Design review of the part shown in the three views and the two pictorial views. Dimensions are in mm from the part's minimum x, y and z. A direction names the side the tool comes from. Round coordinates to 2 decimals unless told otherwise and drop trailing zeros. Write each loop counter-clockwise with the first axis right and the second up, starting at its lowest first coordinate (ties: lowest second). Pieces come first, ordered by that corner, then holes. Notation, with made-up numbers: (45, 89.5) -> (78, 89.5) arc R30 ccw to (78, 118.5) -> close; hole circle Ø2 at (-29.75, 29). An arc over 180 degrees is marked (long way). Return JSON: item names as keys, results as strings. Group by question number.
1. For line 1 along Y through (x, z) = (11.5, 1.75); line 2 along X through (y, z) = (10.25, 6); line 3 along Z through (x, y) = (7, 7), list the stretches that pass through material, from the lowest coordinate up. Write a range as from..to.
2. Mouldability with a two-part tool opening along Y and no side actions: class the marked faces 1, 2 and 3 as pulls with the +Y half, pulls with the -Y half, needs draft (parallel to the pull), parting line crosses it, or undercut.
3. Clearance check with flat-ended pins moving along their axes: P1, Ø6.5, axis at y = 7, z = 6, coming from the +X side; P2, Ø2.5, axis at x = 6.5, z = 5, coming from the -Y side; P3, Ø0.6, axis at y = 13.5, z = 16.5, coming from the +X side. State where each tip first meets the part, or that it passes through.
4. Take a section at B-B, the plane z = 5.25. Write out the cut boundary in (x, y), then the cut area to 3 significant figures.
5. Take a section at A-A, the plane z = 1.5. Write out the cut boundary in (x, y).
6. Take a section at C-C, the plane x = 11.5. Give the number of separate pieces and of enclosed holes in the cut face, then the cut area to 3 significant figures.
7. Tool access review of the marked faces 4, 5 and 6: name each direction out of +Z, -Z, +X, -X, +Y, -Y from which nothing blocks a thin tool from reaching the whole face with its end or side.
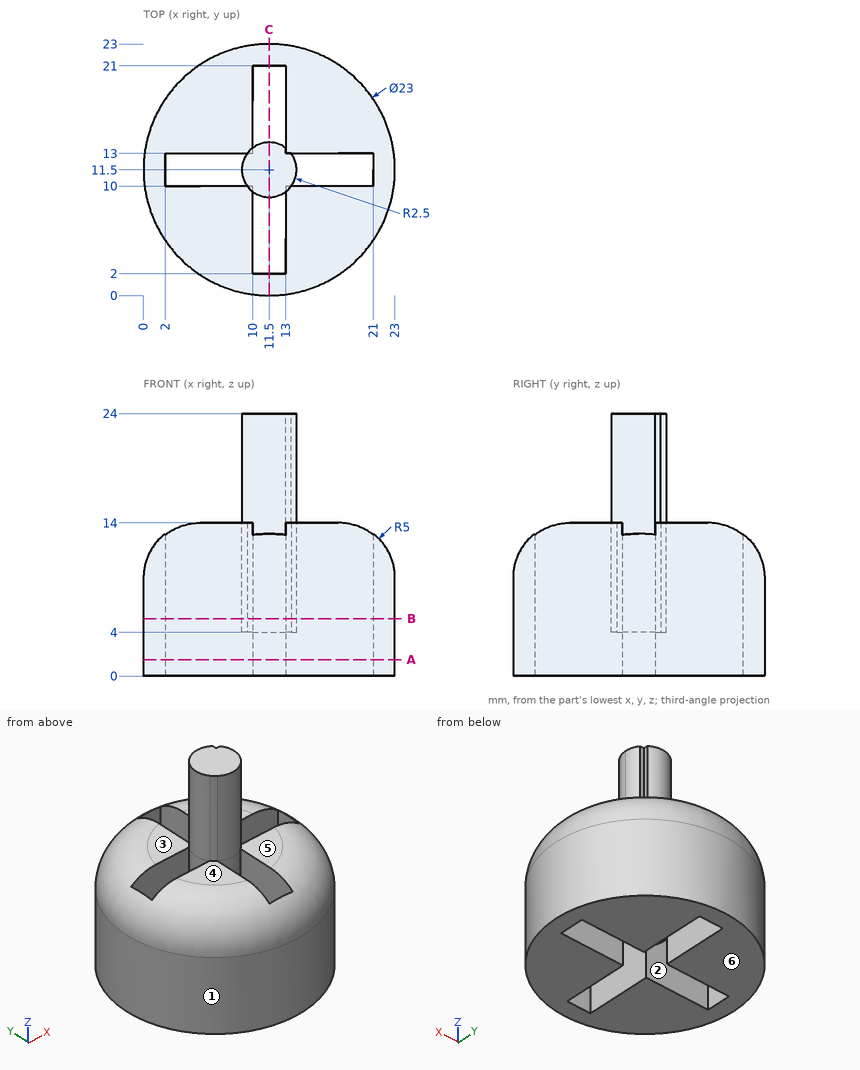
Output:
{
 "1": {"line 1": "y = 0..2, 21..23", "line 2": "x = 0.07..2, 9.33..13.67, 21..22.93", "line 3": "z = 0..14"},
 "2": {"face 1": "parting line crosses it", "face 2": "undercut", "face 3": "needs draft"},
 "3": {"P1": "stops at x = 22.93", "P2": "stops at y = 0.63", "P3": "stops at x = 13"},
 "4": {"outline": "circle Ø23 at (11.5, 11.5); hole (2, 10) -> (9.5, 10) arc R2.5 cw to (9.5, 13) -> (2, 13) -> close; hole (10, 2) -> (13, 2) -> (13, 9.5) arc R2.5 cw to (10, 9.5) -> close; hole (10, 13.5) arc R2.5 cw to (13, 13.5) -> (13, 21) -> (10, 21) -> close; hole (13.5, 10) -> (21, 10) -> (21, 13) -> (13.5, 13) arc R2.5 cw to start", "area": "330 mm^2"},
 "5": {"outline": "circle Ø23 at (11.5, 11.5); hole (2, 10) -> (10, 10) -> (10, 2) -> (13, 2) -> (13, 10) -> (21, 10) -> (21, 13) -> (13, 13) -> (13, 21) -> (10, 21) -> (10, 13) -> (2, 13) -> close"},
 "6": {"separate pieces": "3", "enclosed holes": "0", "area": "147 mm^2"},
 "7": {"face 4": "+Z, -X, -Y", "face 5": "+Z, +X, -Y", "face 6": "-Z, +X, -X, +Y, -Y"}
}
